from build123d import *


with BuildPart() as f1:
    # F0 (on Front) → F1 (revolve)
    with BuildSketch(Plane.XZ):
        with BuildLine():
            Line((-2.5, 4.984315), (-2.5, 7.25))
            Line((-2.5, 7.25), (-4, 7.25))
            Line((-4, 7.25), (-4, 6.45))
            Line((-4, 6.45), (-3.3, 5.914898))
            Line((-3.3, 5.914898), (-3.3, 4.75))
            Line((-3.3, 4.75), (-7.555127, 0.494873))
            ThreePointArc((-7.555127, 0.494873), (-7.76011, 0), (-7.555127, -0.494873))
            Line((-7.555127, -0.494873), (-3.3, -4.75))
            Line((-3.3, -4.75), (-3.3, -6.45))
            Line((-3.3, -6.45), (-4, -6.45))
            Line((-4, -6.45), (-4, -7.25))
            Line((-4, -7.25), (-2.5, -7.25))
            Line((-2.5, -7.25), (-2.5, -4.984315))
            Line((-2.5, -4.984315), (-6.989442, -0.494872))
            ThreePointArc((-6.989442, -0.494872), (-7.194425, 0), (-6.989442, 0.494872))
            Line((-6.989442, 0.494872), (-2.5, 4.984315))
        make_face()
    revolve(axis=Axis((0, 0, -0.799421), (0, 0, -1)))


solid = f1.part
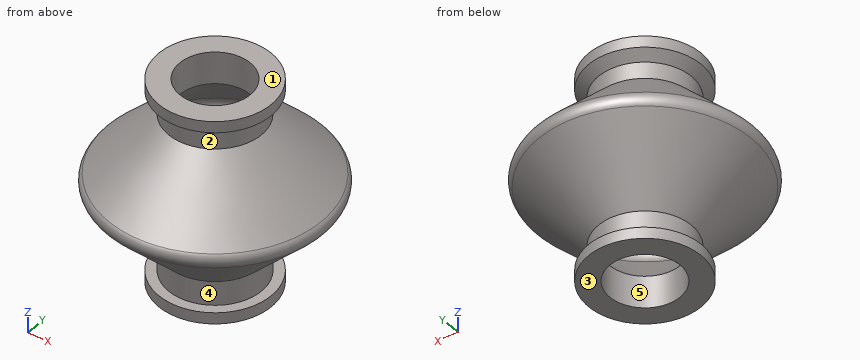
Verification items for the finished model (mm, model axes). Face numbers are marked on the shaded views. A direction names the side the tool comes from. Give positions to 0.01 mm unless a question says otherwise; leave off trailing zeros. Write each loop counter-clockwise with the first axis right and the second up, starting at its lowest first coordinate (ties: lowest second). Pieces come first, ordered by that corner, then holes.
(1) Access from +Z, -Z, +X, -X, +Y, -Y to the whole of each face (thin tool, end or side, straight path). Record for the marked faces 4 and 5.
(2) Gauge pin test, flat ends, axial feed: pin 1 (1.5 mm diameter, centred on x = 3.5, z = 3.5, fed in from -Y); pin 2 (3 mm diameter, centred on x = 3.5, y = 5.5, fed in from +Z); pin 3 (1.5 mm diameter, centred on x = -0.5, z = -3, fed in from -Y); pin 4 (4 mm diameter, centred on x = 0, y = 0, fed in from -Z). Record the tip position at first contact, or that the pin passes through.
(3) Mould release check, pull along Z, two halves, no side actions. Record for the marked faces 1, 2 and 3: +Z half, -Z half, draft (parallel to the pull), parting line (faces both ways), or undercut.
(4) Cross-section at C-C (z = 5.5). Enter the section's corners in (x, y), plus the area to 3 significant figures.
(5) Material ranges on line 1 (Y direction, x = 0, z = 5.5); line 2 (Z direction, x = 3.25, y = -1.75); line 3 (Z direction, x = -3.25, y = -2), recorded low to high.
(6) Cross-section at D-D (z = 0). Enter the section's corners in (x, y), plus the area to 3 significant figures.
Worked out:
1. face 4: none
1. face 5: +Z, -Z
2. pin 1: stops at y = -4.16
2. pin 2: stops at z = 3.03
2. pin 3: stops at y = -5.78
2. pin 4: passes through
3. face 1: +Z half
3. face 2: undercut
3. face 3: -Z half
4. outline: circle Ø6.6 at (0, 0); hole circle Ø5 at (0, 0)
4. area: 14.6 mm2
5. line 1: y = -3.3 to -2.5, 2.5 to 3.3
5. line 2: z = -7.25 to -6.45, -4.36 to -3.79, 3.79 to 4.36, 6.21 to 7.25
5. line 3: z = -7.25 to -6.45, -4.23 to -3.67, 3.67 to 4.23, 6.31 to 7.25
6. outline: circle Ø15.52 at (0, 0); hole circle Ø14.39 at (0, 0)
6. area: 26.6 mm2
